from build123d import *

# Parameters (mm, degrees)
BOSS_EXTRUDE1_DEPTH                                 = 32.5
CBORE_FOR_M8_HEX_SOCKET_HEAD_CAP_SCREW1_D           = 9
CBORE_FOR_M8_HEX_SOCKET_HEAD_CAP_SCREW1_CBORE_D     = 15
CBORE_FOR_M8_HEX_SOCKET_HEAD_CAP_SCREW1_CBORE_DEPTH = 8.6
FILLET1_R                                           = 5


with BuildPart() as part:
    # Sketch1 → Boss-Extrude1 (new body, symmetric)
    with BuildSketch(Plane.XY):
        Polygon((-35, 0), (35, 0), (50, 14.424703588), (50, 25), (42.5, 25), (30, 12.5), (-30, 12.5), (-42.5, 25), (-50, 25), (-50, 14.424703588), align=None)
    extrude(amount=BOSS_EXTRUDE1_DEPTH, both=True)

    # Sketch2 → Revolve1 (revolve)
    with BuildSketch(Plane.XY):
        Polygon((23.5, -30), (26.5, -27), (26.5, -18), (20, -18), (20, -10), (26.5, -10), (26.5, 0), (0, 0), (0, -30), align=None)
    revolve(axis=Axis((0, 0, 0), (0, -1, 0)))

    # CBORE for M8 Hex Socket Head Cap Screw1 (through all)
    with Locations(Plane(origin=(16.815959791, -17.486626004, 0), x_dir=(-0.720794011, -0.69314933, 0), z_dir=(0.69314933, -0.720794011, 0))):
        with Locations((-35.632982274, -20), (-35.632982274, 20)):
            cbore_for_m8_hex_socket_head_cap_screw1 = CounterBoreHole(CBORE_FOR_M8_HEX_SOCKET_HEAD_CAP_SCREW1_D / 2, CBORE_FOR_M8_HEX_SOCKET_HEAD_CAP_SCREW1_CBORE_D / 2, CBORE_FOR_M8_HEX_SOCKET_HEAD_CAP_SCREW1_CBORE_DEPTH)

    # Mirror1: CBORE for M8 Hex Socket Head Cap Screw1 across plane
    add(cbore_for_m8_hex_socket_head_cap_screw1.mirror(Plane(origin=(0, 0, 0), x_dir=(0, 0, 1), z_dir=(1, 0, 0))), mode=Mode.SUBTRACT)

    # Fillet1
    fillet1_edges = [part.edges().sort_by_distance(p)[0] for p in [
        (50, 25, 0),
        (-50, 25, 0),
    ]]
    fillet(fillet1_edges, radius=FILLET1_R)


solid = part.part
Input: part model. Units: mm. Frame: model coordinates. A direction names the side the tool comes from. Coordinates: 2 decimals unless noted, no trailing zeros. Order: outer loops, then holes, each group sorted by start corner. A loop starts at its lowest first (then second) coordinate and runs counter-clockwise, first axis right, second up. Notation, with made-up numbers: M 23,68.5 L 62,68.5 A11 cw 62,85.5 Z; hole C 57.5,-9 d8. An arc over 180 degrees is marked long. One line per question, with ' | ' between items.
Item 1: Ray query, line 1 along Z through (x, y) = (42, 15); line 2 along X through (y, z) = (14.5, 2); line 3 along Y through (x, z) = (25, 3). Return the intervals inside material, ascending.
Geometry results:
line 1: z = -32.5 to -25.56, -14.44 to 14.44, 25.56 to 32.5 | line 2: x = -50 to -32, 32 to 50 | line 3: y = -28.32 to -18, -10 to 12.5
Item 2: Section D-D (z = -17). Give the number of separate pieces and of enclosed holes in the cut face, then the cut area to 3 significant figures.
Geometry results:
separate pieces: 3 | enclosed holes: 0 | area: 2,130 mm^2
Item 3: Reachability of faces 5 (the flat face through (-16, 0, 22)), 6 (the flat face through (4, -18, 20)), 7 (the flat face through (0, 12.5, 0)) from +Z, -Z, +X, -X, +Y, -Y: full face, straight path, thin tool, end or side. Return the list, or none.
Geometry results:
face 5: -Y | face 6: none | face 7: +Z, -Z, +Y
Item 4: Pin query (flat end, axial travel): pin 1 (3 mm diameter, centred on y = 5.5, z = -25, fed in from -X); pin 2 (1.5 mm diameter, centred on y = -8, z = -6, fed in from +X); pin 3 (6 mm diameter, centred on y = 0, z = 1, fed in from +X). Return the tip coordinate at first contact, or that it passes through.
Geometry results:
pin 1: stops at x = -39.24 | pin 2: stops at x = 25.97 | pin 3: stops at x = 38.12
Item 5: Section C-C (y = -12.5). Output: boundary loops of the cut face in (x, z).
Geometry results:
outline: C 0,0 d40
Item 6: Section B-B (x = 0). Output: boundary loops of the cut face in (y, z), then the cut area to 3 significant figures.
Geometry results:
outline: M -30,-23.5 L -27,-26.5 L -18,-26.5 L -18,-20 L -10,-20 L -10,-26.5 L 0,-26.5 L 0,-32.5 L 12.5,-32.5 L 12.5,32.5 L 0,32.5 L 0,26.5 L -10,26.5 L -10,20 L -18,20 L -18,26.5 L -27,26.5 L -30,23.5 Z | area: 2,290 mm^2
Item 7: Draft query along X for faces 1 (the cylindrical face through (40.265, 10.945, -27.436)), 2 (the flat face through (-33.01, 10.02, 19.9)), 3 (the conical face through (-3.08, -29.81, 23.49)), 4 (the flat face through (-42.6, 7.31, 0.45)). Return one class per face: released by +X, released by -X, zero draft, split by the parting line, or undercut.
Geometry results:
face 1: undercut | face 2: undercut | face 3: split by the parting line | face 4: released by -X
Item 8: Section A-A (z = 0). Output: boundary loops of the cut face in (x, y).
Geometry results:
outline: M -50,14.42 L -35,0 L -26.5,0 L -26.5,-10 L -20,-10 L -20,-18 L -26.5,-18 L -26.5,-27 L -23.5,-30 L 23.5,-30 L 26.5,-27 L 26.5,-18 L 20,-18 L 20,-10 L 26.5,-10 L 26.5,0 L 35,0 L 50,14.42 L 50,20 A5 ccw 45,25 L 42.5,25 L 30,12.5 L -30,12.5 L -42.5,25 L -45,25 A5 ccw -50,20 Z
